Build history of the part. All positions in model axes, mm. Face numbers are marked on the shaded views. A direction names the side the tool comes from. Give positions to 0.01 mm unless a question says otherwise; leave off trailing zeros. Write each loop counter-clockwise with the first axis right and the second up, starting at its lowest first coordinate (ties: lowest second). Pieces come first, ordered by that corner, then holes.
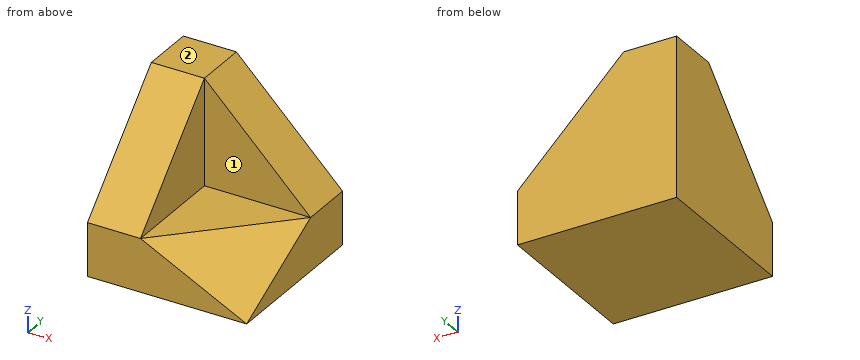
from build123d import *

# Parameters (mm, degrees)
F1_DEPTH = 30
F2_DEPTH = 20
F4_DEPTH = 10.001
F7_DEPTH = 24.4958974278


with BuildPart() as f1:
    # F0 (on Front) → F1 (new body)
    with BuildSketch(Plane.XZ):
        Polygon((0, 30), (0, 0), (30, 0), (30, 10), (10, 10), (10, 30), align=None)
        Polygon((10, 10), (30, 10), (10, 30), align=None)
    extrude(amount=-F1_DEPTH)

    # F0 (on Front) → F2 (cut)
    with BuildSketch(Plane.XZ):
        Polygon((10, 10), (30, 10), (10, 30), align=None)
    extrude(amount=-F2_DEPTH, mode=Mode.SUBTRACT)

    # F3 (on face) → F4 (cut, through all)
    with BuildSketch(Plane.YZ.offset(10)):
        Polygon((0, 10), (20, 30), (0, 30), align=None)
    extrude(amount=-F4_DEPTH, mode=Mode.SUBTRACT)

    # F6 (on 3pt) → F7 (cut, through all)
    with BuildSketch(Plane(origin=(5, -5, 10), x_dir=(0.9128709292, 0.1825741858, -0.3651483717), z_dir=(-0.4082482905, 0.4082482905, -0.8164965809))):
        Polygon((5.4772255751, -4.472135955), (27.3861278753, -22.360679775), (27.3861278753, 0), align=None)
    extrude(amount=-F7_DEPTH, mode=Mode.SUBTRACT)


solid = f1.part
1. Drill centre lines: line 1 along Z through (x, y) = (14, 9); line 2 along Y through (x, z) = (16.5, 23). Where is each one in solid material? Low to high.
2. Saw through at A-A on x = 23. Give the cut face in (y, z), plus the area to 3 significant figures.
3. 3-axis set-ups, long thin cutter, end or side, ignore diameter. For the marked faces 1 and 2: which of +Z, -Z, +X, -X, +Y, -Y reach the whole face in a straight line?
4. Saw through at B-B on y = 19. Give the cut face in (x, z), plus the area to 3 significant figures.
5. Saw through at C-C on z = 18. Give the cut face in (x, y).
6. Saw through at D-D on z = 9. Give the cut face in (x, y), plus the area to 3 significant figures.
7. Drop flat-ended pins along their axis: pin 1 (6 mm diameter, centred on x = 19, y = 7, fed in from +Z); pin 2 (10 mm diameter, centred on x = 9, z = 22, fed in from -Y); pin 3 (1 mm diameter, centred on y = 21, z = 9, fed in from -X); pin 4 (6 mm diameter, centred on x = 22.5, z = 21.5, fed in from -Y). Give the stop position or say it passes through.
Outcome:
1. line 1: z = 0 to 10
1. line 2: y = 20 to 30
2. outline: (0, 0) - (30, 0) - (30, 17) - (20, 17) - (20, 10) - (13, 10) - (0, 3.5) - close
2. area: 328 mm2
3. face 1: +Z, +X, -Y
3. face 2: +Z, +X, -X, +Y, -Y
4. outline: (0, 0) - (30, 0) - (30, 9.5) - (29, 10) - (10, 10) - (10, 29) - (0, 29) - close
4. area: 490 mm2
5. outline: (0, 8) - (10, 8) - (10, 20) - (22, 20) - (22, 30) - (0, 30) - close
6. outline: (0, 0) - (12, 0) - (30, 18) - (30, 30) - (0, 30) - close
6. area: 738 mm2
7. pin 1: stops at z = 10
7. pin 2: stops at y = 7
7. pin 3: stops at x = 0
7. pin 4: stops at y = 20
